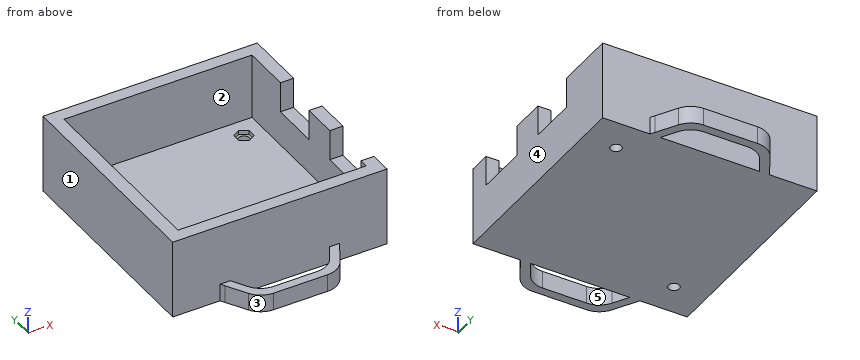
from build123d import *

# Parameters (mm, degrees)
SKETCH_1_W          = 49
SKETCH_1_H          = 50
EXTRUDE_1_DEPTH     = 10
SKETCH_3_W          = 43
SKETCH_3_H          = 44
CUT_EXTRUDE_1_DEPTH = 7
CUT_EXTRUDE_2_DEPTH = 1
SKETCH_5_R          = 1.25
CUT_EXTRUDE_3_DEPTH = 3
SKETCH_7_W          = 8
SKETCH_7_H          = 50
EXTRUDE_2_DEPTH     = 3
SKETCH_8_W          = 7
SKETCH_8_H          = 12
SKETCH_8_H_2        = 11
CUT_EXTRUDE_5_DEPTH = 3
EXTRUDE_3_DEPTH     = 8
EXTRUDE_4_DEPTH     = 4


with BuildPart() as part:
    # 草图1 → 凸台-拉伸1 (new body)
    with BuildSketch(Plane.XY):
        Rectangle(SKETCH_1_W, SKETCH_1_H)
    extrude(amount=EXTRUDE_1_DEPTH)

    # 草图3 → 切除-拉伸1 (cut)
    with BuildSketch(Plane.XY.offset(10)):
        Rectangle(SKETCH_3_W, SKETCH_3_H)
    extrude(amount=-CUT_EXTRUDE_1_DEPTH, mode=Mode.SUBTRACT)

    # 草图4 → 切除-拉伸2 (cut)
    with BuildSketch(Plane.XY.offset(3)):
        Polygon((17, 15.479274058), (18.75, 16.489637029), (18.75, 18.510362971), (17, 19.520725942), (15.25, 18.510362971), (15.25, 16.489637029), align=None)
        Polygon((-17, -19.520725942), (-15.25, -18.510362971), (-15.25, -16.489637029), (-17, -15.479274058), (-18.75, -16.489637029), (-18.75, -18.510362971), align=None)
    extrude(amount=-CUT_EXTRUDE_2_DEPTH, mode=Mode.SUBTRACT)

    # 草图5 → 切除-拉伸3 (cut)
    with BuildSketch(Plane.XY.offset(2)):
        with Locations((-17, -17.5)):
            Circle(SKETCH_5_R)
        with Locations((17, 17.5)):
            Circle(SKETCH_5_R)
    extrude(amount=-CUT_EXTRUDE_3_DEPTH, mode=Mode.SUBTRACT)

    # 草图7 → 凸台-拉伸2 (add)
    with BuildSketch(Plane(origin=(24.5, 0, 0), x_dir=(0, 0, -1), z_dir=(1, 0, 0))):
        with Locations((-14, 0)):
            Rectangle(SKETCH_7_W, SKETCH_7_H)
    extrude(amount=-EXTRUDE_2_DEPTH)

    # 草图8 → 切除-拉伸5 (cut)
    with BuildSketch(Plane(origin=(24.5, 0, 0), x_dir=(0, 0, -1), z_dir=(1, 0, 0))):
        with Locations((-14.5, -14)):
            Rectangle(SKETCH_8_W, SKETCH_8_H)
        with Locations((-14.5, 5.5)):
            Rectangle(SKETCH_8_W, SKETCH_8_H_2)
    extrude(amount=-CUT_EXTRUDE_5_DEPTH, mode=Mode.SUBTRACT)

    # 草图9 → 凸台-拉伸3 (add)
    with BuildSketch(Plane.XY.offset(10)):
        Polygon((-24.5, -25), (21.5, -25), (21.5, -22), (-21.5, -22), (-21.5, 22), (21.5, 22), (21.5, 25), (-24.5, 25), align=None)
    extrude(amount=EXTRUDE_3_DEPTH)

    # 草图11 → 凸台-拉伸4 (add)
    with BuildSketch(Plane(origin=(0, 0, 0), x_dir=(-1, 0, 0), z_dir=(0, 0, -1))):
        with BuildLine():
            Line((-13.660254038, -25), (-11.350852961, -25))
            Line((-11.350852961, -25), (-9.330127019, -28.5))
            ThreePointArc((-9.330127019, -28.5), (-7.5, -30.330127019), (-5, -31))
            Line((-5, -31), (5, -31))
            ThreePointArc((5, -31), (7.5, -30.330127019), (9.330127019, -28.5))
            Line((9.330127019, -28.5), (11.350852961, -25))
            Line((11.350852961, -25), (13.660254038, -25))
            Line((13.660254038, -25), (13.082903769, -26))
            Line((13.082903769, -26), (10.484827557, -30.5))
            ThreePointArc((10.484827557, -30.5), (8.654700538, -32.330127019), (6.154700538, -33))
            Line((6.154700538, -33), (-6.154700538, -33))
            ThreePointArc((-6.154700538, -33), (-8.654700538, -32.330127019), (-10.484827557, -30.5))
            Line((-10.484827557, -30.5), (-13.082903769, -26))
            Line((-13.082903769, -26), (-13.660254038, -25))
        make_face()
    extrude_4 = extrude(amount=-EXTRUDE_4_DEPTH)

    # 镜向1: 凸台-拉伸4 across plane
    add(extrude_4.mirror(Plane.ZX))


solid = part.part
Work out the finished part from the listing and answer in its coordinate system (mm). Face numbers are marked on the shaded views. A direction names the side the tool comes from. Give positions to 0.01 mm unless a question says otherwise; leave off trailing zeros. Write each loop counter-clockwise with the first axis right and the second up, starting at its lowest first coordinate (ties: lowest second). Pieces come first, ordered by that corner, then holes. Notation, with made-up numbers: (45.5, 28.25) - (94.5, 28.25) arc R11 cw to (94.5, 40.25) - close; hole circle Ø11 at (19, 8). An arc over 180 degrees is marked (long way). One line per item, written item: value. Start each with the question number.
1. For the marked faces 1 and 2, determine the directions among +Z, -Z, +X, -X, +Y, -Y from which every point of the face is accessible in a straight line to the end or side of a thin tool.
2. Given pin 1 (2.5 mm diameter, centred on x = 23, y = -13.5, fed in from +Z); pin 2 (1.5 mm diameter, centred on x = -17, z = 14, fed in from -Y); pin 3 (3.5 mm diameter, centred on x = 23, z = 13, fed in from +Y), each flat-ended and moving along its own axis, determine where each tip first touches the part or whether it passes through.
3. Find section A-A (z = 12.75). Write down the section's boundary in (x, y), then the cut area to 3 significant figures.
4. For a pull along X with two mould halves and no side action, classify the marked faces 3, 4 and 5 as +X half, -X half, draft (parallel to the pull), parting line (faces both ways), or undercut.
5. Find section B-B (x = -2). Write down the section's boundary in (y, z).
6. Consider probe 1 along Y at (x, z) = (17, 0.4); probe 2 along Y at (x, z) = (0, 11.5); probe 3 along X at (y, z) = (-6, 4). Determine where each line is inside the solid, lowest interval first.
7. Find section C-C (y = 17.5). Write down the section's boundary in (x, z).
8. Find section D-D (z = 6.5). Write down the section's boundary in (x, y).
Geometry results:
1. face 1: +Z, -Z, -X, +Y, -Y
1. face 2: +Z
2. pin 1: z = 11
2. pin 2: y = -25
2. pin 3: y = 25
3. outline: (-24.5, -25) - (24.5, -25) - (24.5, -20) - (21.5, -20) - (21.5, -22) - (-21.5, -22) - (-21.5, 22) - (21.5, 22) - (21.5, 11) - (24.5, 11) - (24.5, 25) - (-24.5, 25) - close; (21.5, -8) - (24.5, -8) - (24.5, 0) - (21.5, 0) - close
3. area: 489 mm2
4. face 3: -X half
4. face 4: +X half
4. face 5: undercut
5. outline: (-33, 0) - (-31, 0) - (-31, 4) - (-33, 4) - close; (-25, 0) - (25, 0) - (25, 18) - (22, 18) - (22, 3) - (-22, 3) - (-22, 18) - (-25, 18) - close; (31, 0) - (33, 0) - (33, 4) - (31, 4) - close
6. probe 1: -25 to 16.25, 18.75 to 25
6. probe 2: -25 to -22, 22 to 25
6. probe 3: -24.5 to -21.5, 21.5 to 24.5
7. outline: (-24.5, 0) - (15.75, 0) - (15.75, 2) - (15.25, 2) - (15.25, 3) - (-21.5, 3) - (-21.5, 18) - (-24.5, 18) - close; (18.25, 0) - (24.5, 0) - (24.5, 18) - (21.5, 18) - (21.5, 3) - (18.75, 3) - (18.75, 2) - (18.25, 2) - close
8. outline: (-24.5, -25) - (24.5, -25) - (24.5, 25) - (-24.5, 25) - close; hole (-21.5, -22) - (21.5, -22) - (21.5, 22) - (-21.5, 22) - close
